Autodesk Inventor part; units mm, degrees
ref_plane "YZ Plane" through (0, 0, 0) normal (1, 0, 0) x (0, 1, 0)
ref_plane "XZ Plane" through (0, 0, 0) normal (0, 1, 0) x (-1, 0, 0)
ref_plane "XY Plane" through (0, 0, 0) normal (0, 0, 1) x (1, 0, 0)
sketch "Sketch1" plane through (0, 0, 0) normal (0, 0, 1) x (1, 0, 0)
  line L0 (-125, -75) -> (125, -75)
  line L1 (125, -75) -> (125, 75)
  line L2 (125, 75) -> (-125, 75)
  line L3 (-125, 75) -> (-125, -75)
  line L4 (-125, -75) -> (125, 75) construction
  line L5 (125, -75) -> (-125, 75) construction
  point P0 (0, 0)
  dimension "d0" = 150
  dimension "d1" = 250
extrude "Extrusion1" add sketch "Sketch1" along normal blind 3
sketch "Sketch2" plane through (0, 0, 3) normal (0, 0, 1) x (1, 0, 0)
  line L0 (125, -75) -> (125, 75) construction
  line L1 (125, 75) -> (-125, 75) construction
  line L2 (-125, 75) -> (-125, -75) construction
  line L3 (-125, -75) -> (125, -75) construction
  line L4 (-125, -36) -> (-105, -36)
  line L5 (-105, -36) -> (-105, -55)
  line L6 (-105, -55) -> (-86, -55)
  line L7 (-86, -55) -> (-86, -75)
  line L8 (-125, -75) -> (125, -75) construction
  line L9 (-125, 75) -> (-125, -75) construction
  line L10 (-125, -36) -> (-125, -75)
  line L11 (-86, -75) -> (-125, -75)
  line L12 (-125, 33) -> (-101, 33)
  line L13 (-101, 33) -> (-101, -16)
  line L14 (-101, -16) -> (-125, -16)
  line L15 (-125, -16) -> (-125, 33)
  line L16 (65, -75) -> (75, -75)
  line L17 (75, -75) -> (75, -45)
  line L18 (75, -45) -> (65, -45)
  line L19 (65, -45) -> (65, -75)
  line L20 (125, 75) -> (-125, 75)
  line L21 (-125, 75) -> (-101, 75)
  line L22 (-101, 75) -> (-101, 53)
  line L23 (-101, 53) -> (-125, 53)
  line L24 (-125, 53) -> (-125, 75)
  point P0 (0, 0)
  dimension "d4" = 39
  dimension "d5" = 39
  dimension "d6" = 20
  dimension "d7" = 20
  dimension "d9" = 24
  dimension "d11" = 20
  dimension "d13" = 10
  dimension "d14" = 30
  dimension "d36" = 50
  dimension "d37" = 22
  dimension "d39" = 42
extrude "Extrusion2" cut sketch "Sketch2" against normal blind 3
sketch "Sketch3" plane through (0, 0, 3) normal (0, 0, 1) x (1, 0, 0)
  circle A0 centre (-115, 43) radius 2.25
  circle A1 centre (-115, -26) radius 2.25
  circle A2 centre (115, 65) radius 2.25
  circle A3 centre (115, -65) radius 2.25
  circle A4 centre (-76, -65) radius 2.25
  line L0 (125, 75) -> (-125, 75)
  line L1 (-125, 75) -> (-125, 33)
  line L2 (-125, -16) -> (-125, -36)
  line L3 (-125, -36) -> (-105, -36)
  line L4 (-86, -75) -> (65, -75)
  line L5 (-86, -55) -> (-86, -75)
  line L6 (75, -75) -> (125, -75)
  line L7 (125, -75) -> (125, 75)
  line L8 (-125, 53) -> (-101, 53)
  point P0 (0, 0)
  dimension "d17" = 4.5
  dimension "d18" = 4.5
  dimension "d19" = 4.5
  dimension "d20" = 4.5
  dimension "d21" = 4.5
  dimension "d23" = 10
  dimension "d24" = 10
  dimension "d25" = 10
  dimension "d26" = 10
  dimension "d27" = 10
  dimension "d28" = 10
  dimension "d29" = 10
  dimension "d30" = 10
  dimension "d31" = 10
  dimension "d38" = 10
extrude "Extrusion3" cut sketch "Sketch3" against normal through all
fillet "Fillet1" radius 2 14 edges at (125, 75, 1.5) (125, -75, 1.5) (-86, -75, 1.5) (-86, -55, 1.5) (-105, -55, 1.5) (-105, -36, 1.5) (-125, -36, 1.5) (-125, -16, 1.5) (-101, -16, 1.5) (-101, 33, 1.5) (-125, 33, 1.5) (-125, 53, 1.5) (-101, 53, 1.5) (-101, 75, 1.5)
fillet "Fillet1" radius 5 2 edges at (65, -45, 1.5) (75, -45, 1.5)
sketch "Sketch4" plane through (0, 0, 3) normal (0, 0, 1) x (1, 0, 0)
  arc A0 (-99, 75) -> (-101, 73) centre (-99, 73) ccw
  line L0 (-101, 73) -> (-101, 55)
  arc A1 (-103, 53) -> (-101, 55) centre (-103, 55) ccw
  line L1 (-103, 53) -> (-123, 53)
  arc A2 (-123, 53) -> (-125, 51) centre (-123, 51) ccw
  line L2 (-125, 51) -> (-125, 35)
  arc A3 (-125, 35) -> (-123, 33) centre (-123, 35) ccw
  line L3 (-123, 33) -> (-103, 33)
  arc A4 (-101, 31) -> (-103, 33) centre (-103, 31) ccw
  line L4 (-101, 31) -> (-101, -14)
  arc A5 (-103, -16) -> (-101, -14) centre (-103, -14) ccw
  line L5 (-103, -16) -> (-123, -16)
  arc A6 (-123, -16) -> (-125, -18) centre (-123, -18) ccw
  line L6 (-125, -18) -> (-125, -34)
  arc A7 (-125, -34) -> (-123, -36) centre (-123, -34) ccw
  line L7 (-123, -36) -> (-107, -36)
  arc A8 (-105, -38) -> (-107, -36) centre (-107, -38) ccw
  line L8 (-105, -38) -> (-105, -53)
  arc A9 (-105, -53) -> (-103, -55) centre (-103, -53) ccw
  line L9 (-103, -55) -> (-88, -55)
  arc A10 (-86, -57) -> (-88, -55) centre (-88, -57) ccw
  line L10 (-86, -57) -> (-86, -73)
  arc A11 (-86, -73) -> (-84, -75) centre (-84, -73) ccw
  line L11 (-84, -75) -> (65, -75)
  line L12 (65, -75) -> (65, -50)
  arc A12 (75, -50) -> (65, -50) centre (70, -50) ccw
  line L13 (75, -50) -> (75, -75)
  line L14 (75, -75) -> (123, -75)
  arc A13 (123, -75) -> (125, -73) centre (123, -73) ccw
  line L15 (125, -73) -> (125, 73)
  arc A14 (125, 73) -> (123, 75) centre (123, 73) ccw
  line L16 (123, 75) -> (-99, 75)
  circle A15 centre (-115, 43) radius 2.25
  circle A16 centre (115, 65) radius 2.25
  circle A17 centre (-115, -26) radius 2.25
  circle A18 centre (115, -65) radius 2.25
  circle A19 centre (-76, -65) radius 2.25
  point P0 (0, 0)
equation "\"d5\" = d4"
equation "\"d18\" = d17"
equation "\"d19\" = d17"
equation "\"d20\" = d17"
equation "\"d21\" = d17"
equation "\"d24\" = d23"
equation "\"d25\" = d23"
equation "\"d26\" = d25"
equation "\"d27\" = d25"
equation "\"d28\" = d26"
equation "\"d29\" = d26"
equation "\"d30\" = d23"
equation "\"d31\" = d23"
equation "\"d38\" = d23"
properties part number "SideAcrylicSheet"
Work out the finished part from the listing and answer in its coordinate system (mm). A direction names the side the tool comes from. Round coordinates to 2 decimals unless told otherwise and drop trailing zeros. Write each loop counter-clockwise with the first axis right and the second up, starting at its lowest first coordinate (ties: lowest second). Pieces come first, ordered by that corner, then holes.
1) The mould has two halves that part along Y. Classify faces 3 (the flat face through (-2, 1, 0)), 4 (the cylindrical face through (73, -46, 1)), 5 (the cylindrical face through (117.08, 64.14, 1.52)): pulls with the +Y half, pulls with the -Y half, needs draft (parallel to the pull), parting line crosses it, or undercut.
2) A cutting plane is placed at A-A (z = 0.8). Give the number of separate pieces and of enclosed holes in the cut face, plus the area to 3 significant figures.
3) A cutting plane is placed at B-B (y = -3.5). Give the vertices of the cut face in (x, z).
4) Given pin 1 Ø1.5 at (x, z) = (-113, 2) entering from +Y; pin 2 Ø1.5 at (x, z) = (-112.5, 2) entering from -Y; pin 3 Ø0.9 at (y, z) = (-58, 2) entering from -X, each flat-ended and moving along its own axis, determine where each tip first touches the part or whether it passes through.
5) A tool of negligible diameter and unlimited length cuts with its end or side. For faces 1 (the cylindrical face through (66, -47, 1)), 2 (the cylindrical face through (-112.854, 43.676, 1.521)), from which of +Z, -Z, +X, -X, +Y, -Y can it reach the whole face along a straight path? Write none if from no direction.
6) Straight lines are drawn through the part: line 1 (Y direction, x = 115, z = 2.3); line 2 (Y direction, x = -115, z = 0.9); line 3 (Y direction, x = -76, z = 1.5). For each, find the intervals that lie inside material, in ascending order.
Completed:
1. face 3: needs draft
1. face 4: pulls with the -Y half
1. face 5: undercut
2. separate pieces: 1
2. enclosed holes: 5
2. area: 34,300 mm2
3. outline: (-101, 0) - (125, 0) - (125, 3) - (-101, 3) - close
4. pin 1: stops at y = 53
4. pin 2: stops at y = -36
4. pin 3: stops at x = -86
5. face 1: +Z, -Z, -Y
5. face 2: +Z, -Z
6. line 1: y = -75 to -67.25, -62.75 to 62.75, 67.25 to 75
6. line 2: y = -36 to -28.25, -23.75 to -16, 33 to 40.75, 45.25 to 53
6. line 3: y = -75 to -67.25, -62.75 to 75
